from build123d import *

# Parameters (mm, degrees)
SKETCH1_R              = 3.048
BOSS_EXTRUDE1_DEPTH    = 3.048
SKETCH2_W              = 28.575
SKETCH2_H              = 3.048
BOSS_EXTRUDE2_DEPTH    = 17.78
CUT_EXTRUDE1_DEPTH     = 45.290237175
FILLET1_R              = 3.81
CONVERT_SOLID1_START   = -28.575
CONVERT_SOLID1_DEPTH   = 28.575
CONVERT_SOLID1_2_DEPTH = 28.575


# Read off the part's stored shape, not the designer's step: Convert-Solid1
with BuildPart() as part:
    # Sketch1 → Boss-Extrude1 (new body)
    with BuildSketch(Plane(origin=(0, 0, 0), x_dir=(0, 0, -1), z_dir=(1, 0, 0))):
        with BuildLine():
            Line((28.575, 6.35), (13.771011503, 26.59571692))
            ThreePointArc((13.771011503, 26.59571692), (5.254234548, 29.341449028), (0, 22.098))
            Line((0, 22.098), (0, 0))
            Line((0, 0), (28.575, 0))
            Line((28.575, 0), (28.575, 6.35))
        make_face()
        with Locations(Location((7.62, 22.098, 0), (0, 0, 180))):
            Circle(SKETCH1_R, mode=Mode.SUBTRACT)
    extrude(amount=BOSS_EXTRUDE1_DEPTH)

    # Sketch2 → Boss-Extrude2 (add)
    with BuildSketch(Plane(origin=(3.048, 0, 0), x_dir=(0, 0, -1), z_dir=(1, 0, 0))):
        with Locations((14.2875, 1.524)):
            Rectangle(SKETCH2_W, SKETCH2_H)
    extrude(amount=BOSS_EXTRUDE2_DEPTH)

    # Sketch3 → Cut-Extrude1 (cut, through all)
    with BuildSketch(Plane(origin=(0, 3.048, 0), x_dir=(1, 0, 0), z_dir=(0, 1, 0))):
        with BuildLine():
            Line((8.128, 4.953), (8.128, 0))
            Line((8.128, 0), (14.478, 0))
            Line((14.478, 0), (14.478, 4.953))
            ThreePointArc((14.478, 4.953), (11.303, 8.128), (8.128, 4.953))
        make_face()
        with BuildLine():
            Line((8.128, 28.575), (8.128, 23.622))
            ThreePointArc((8.128, 23.622), (11.303, 20.447), (14.478, 23.622))
            Line((14.478, 23.622), (14.478, 28.575))
            Line((14.478, 28.575), (8.128, 28.575))
        make_face()
    extrude(amount=-CUT_EXTRUDE1_DEPTH, mode=Mode.SUBTRACT)

    # Fillet1
    fillet1_edges = [part.edges().sort_by_distance(p)[0] for p in [
        (20.828, 1.524, 0),
        (20.828, 1.524, -28.575),
    ]]
    fillet(fillet1_edges, radius=FILLET1_R)

    # Convert-Solid1 outline → Convert-Solid1 (cut)
    with BuildSketch(Plane.XY.offset(CONVERT_SOLID1_START)):
        with BuildLine():
            Line((0, 0), (4.548, 0))
            ThreePointArc((4.548, 0), (1.332078359, 1.332078359), (0, 4.548))
            Line((0, 4.548), (0, 0))
        make_face()
    extrude(amount=CONVERT_SOLID1_DEPTH, mode=Mode.SUBTRACT)

    # Convert-Solid1 2 outline → Convert-Solid1 2 (add)
    with BuildSketch(Plane.XY.offset(CONVERT_SOLID1_START)):
        with BuildLine():
            Line((3.048, 3.048), (4.548, 3.048))
            ThreePointArc((4.548, 3.048), (3.487339828, 3.487339828), (3.048, 4.548))
            Line((3.048, 4.548), (3.048, 3.048))
        make_face()
    extrude(amount=CONVERT_SOLID1_2_DEPTH)


solid = part.part
Source: CAD feature listing. Evaluate the final solid. Frame: model axes, mm. A direction names the side the tool comes from. Round coordinates to 2 decimals unless told otherwise and drop trailing zeros. Write each loop counter-clockwise with the first axis right and the second up, starting at its lowest first coordinate (ties: lowest second). Pieces come first, ordered by that corner, then holes. Notation, with made-up numbers: M 79,67 L 122,67 A21 ccw 122,100 Z; hole C -15.5,-9.5 d1. An arc over 180 degrees is marked long. One line per item, written item: value. Start each with the question number.
Item 1: Section query C-C (y = 2.5). Return the cut outline in (x, z) (3 decimals), plus the area to 3 significant figures.
Item 2: Mould query, pull axis X, two halves, no side actions, for faces 5 (the cylindrical face through (19.74, 1.55, -27.43)), 6 (the cylindrical face through (1.5, 29.38, -5.38)), 7 (the flat face through (8.128, 2, -3)). Classes: pulls with the +X half, pulls with the -X half, needs draft (parallel to the pull), parting line crosses it, or undercut.
Item 3: Section query B-B (z = -7.62). Return the cut outline in (x, y), plus the area to 3 significant figures.
Item 4: Ray query, L1, parallel to X at y = 9.25, z = -2.5; L2, parallel to Y at x = 0.85, z = -7.62. Return the intervals inside material, ascending. Write a range as from..to.
Item 5: Set-up query: faces 1 (the flat face through (14.478, 2, -26)), 2 (the flat face through (13, 3.048, -14)), 3 (the flat face through (20.828, 2, -14)), 4 (the flat face through (14.478, 2, -2)). Return all of +Z, -Z, +X, -X, +Y, -Y with unobstructed straight access to the full face (end or side cutting, diameter ignored); none if empty.
Item 6: Pin query (flat end, axial travel): pin 1 (0.9 mm diameter, centred on y = 1.5, z = -25.5, fed in from -X); pin 2 (1.5 mm diameter, centred on x = 17.5, z = -21.5, fed in from +Y); pin 3 (5.5 mm diameter, centred on y = 22.098, z = -7.62, fed in from +X); pin 4 (2.5 mm diameter, centred on y = 2, z = -3.5, fed in from -X). Return the tip coordinate at first contact, or that it passes through.
Item 7: Section query A-A (z = -22.25). Return the cut outline in (x, y), plus the area to 3 significant figures.
Item 8: Section query D-D (z = -19.25). Return the cut outline in (x, y), plus the area to 3 significant figures.
Result set:
1. outline: M 0.487,-28.575 L 8.128,-28.575 L 8.128,-23.622 A3.175 cw 14.478,-23.622 L 14.478,-28.575 L 17.018,-28.575 A3.81 ccw 20.828,-24.765 L 20.828,-3.81 A3.81 ccw 17.018,0 L 14.478,0 L 14.478,-4.953 A3.175 cw 8.128,-4.953 L 8.128,0 L 0.487,0 Z
1. area: 480 mm²
2. face 5: pulls with the +X half
2. face 6: needs draft
2. face 7: undercut
3. outline: M 0,4.55 A4.55 ccw 4.55,0 L 9.58,0 L 9.58,3.05 L 4.55,3.05 A1.5 cw 3.05,4.55 L 3.05,19.05 L 0,19.05 Z; M 0,25.15 L 3.05,25.15 L 3.05,29.72 L 0,29.72 Z; M 13.03,0 L 20.83,0 L 20.83,3.05 L 13.03,3.05 Z
3. area: 112 mm²
4. L1: x = 0..3.05
4. L2: y = 1.9..19.05, 25.15..29.72
5. face 1: -Z, +Y, -Y
5. face 2: +Z, -Z, +X, +Y
5. face 3: +Z, -Z, +X, +Y, -Y
5. face 4: +Z, +Y, -Y
6. pin 1: stops at x = 0.82
6. pin 2: stops at y = 3.05
6. pin 3: passes through
6. pin 4: stops at x = 0.19
7. outline: M 0,4.55 A4.55 ccw 4.55,0 L 8.44,0 L 8.44,3.05 L 4.55,3.05 A1.5 cw 3.05,4.55 L 3.05,15 L 0,15 Z; M 14.17,0 L 20.83,0 L 20.83,3.05 L 14.17,3.05 Z
7. area: 78.5 mm²
8. outline: M 0,4.55 A4.55 ccw 4.55,0 L 20.83,0 L 20.83,3.05 L 4.55,3.05 A1.5 cw 3.05,4.55 L 3.05,19.1 L 0,19.1 Z
8. area: 108 mm²
